Check sheet for the modelled part. Datum: model origin and axes. Units: mm. A direction names the side the tool comes from. Round coordinates to 2 decimals unless told otherwise and drop trailing zeros. Loops run counter-clockwise (first coordinate to the right, second up) from the corner with the lowest first, then second, coordinate; pieces in that order, holes last. Notation, with made-up numbers: (65, -24.75) -> (90, -24.75) arc R33 cw to (90, 7.25) -> close; hole circle Ø6 at (62, 41.5). An arc over 180 degrees is marked (long way). One line per question, with ' | ' between items.
```python
from build123d import *

# Parameters (mm, degrees)
SKETCH_1_R                   = 8
EXTRUDE_1_DEPTH              = 6
CUT_EXTRUDE_1_DEPTH          = 3.2
HOLE_WIZARD_M2_1_D           = 2.4
HOLE_WIZARD_M2_1_CBORE_D     = 4.2
HOLE_WIZARD_M2_1_CBORE_DEPTH = 2.5
PATTERN_CIRCULAR_1_COUNT     = 4
HOLE_WIZARD_M4_1_D           = 5


with BuildPart() as part:
    # ｽｹｯﾁ1 → ﾎﾞｽ - 押し出し1 (new body)
    with BuildSketch(Plane.XY):
        Circle(SKETCH_1_R)
    extrude(amount=EXTRUDE_1_DEPTH)

    # ｽｹｯﾁ2 → ｶｯﾄ - 押し出し1 (cut)
    with BuildSketch(Plane.XY.offset(6)):
        Polygon((4.070319398, 0), (2.035159699, 3.525), (-2.035159699, 3.525), (-4.070319398, 0), (-2.035159699, -3.525), (2.035159699, -3.525), align=None)
    extrude(amount=-CUT_EXTRUDE_1_DEPTH, mode=Mode.SUBTRACT)

    # M2 丸平ねじ用座ぐり穴1 (through all)
    with Locations(Plane(origin=(0, 0, 0), x_dir=(-1, 0, 0), z_dir=(0, 0, -1))):
        with Locations((6, 0)):
            hole_wizard_m2_1 = CounterBoreHole(HOLE_WIZARD_M2_1_D / 2, HOLE_WIZARD_M2_1_CBORE_D / 2, HOLE_WIZARD_M2_1_CBORE_DEPTH)

    # 円形ﾊﾟﾀｰﾝ1: M2 丸平ねじ用座ぐり穴1 ×4 about axis
    pattern_circular_1_axis = Axis((0, 0, 0), (0, 0, 1))
    for i in range(1, PATTERN_CIRCULAR_1_COUNT):
        add(hole_wizard_m2_1.rotate(pattern_circular_1_axis, i * 360 / PATTERN_CIRCULAR_1_COUNT), mode=Mode.SUBTRACT)

    # M4 すきま穴1 (through all)
    with Locations(Plane(origin=(0, 0, 0), x_dir=(-1, 0, 0), z_dir=(0, 0, -1))):
        with Locations((0, 0)):
            Hole(HOLE_WIZARD_M4_1_D / 2)


solid = part.part
```
(1) Sectioned sample at B-B, the plane y = 6. Record the cut outline in (x, z).
Answer:
outline: (-5.29, 0) -> (-2.1, 0) -> (-2.1, 2.5) -> (-1.2, 2.5) -> (-1.2, 6) -> (-5.29, 6) -> close; (1.2, 2.5) -> (2.1, 2.5) -> (2.1, 0) -> (5.29, 0) -> (5.29, 6) -> (1.2, 6) -> close
(2) Sectioned sample at C-C, the plane x = -1. Record the cut outline in (y, z) (3 decimals).
Answer:
outline: (-7.937, 0) -> (-7.847, 0) -> (-7.847, 2.5) -> (-6.663, 2.5) -> (-6.663, 6) -> (-7.937, 6) -> close; (-5.337, 2.5) -> (-4.153, 2.5) -> (-4.153, 0) -> (-2.291, 0) -> (-2.291, 2.8) -> (-3.525, 2.8) -> (-3.525, 6) -> (-5.337, 6) -> close; (2.291, 0) -> (4.153, 0) -> (4.153, 2.5) -> (5.337, 2.5) -> (5.337, 6) -> (3.525, 6) -> (3.525, 2.8) -> (2.291, 2.8) -> close; (6.663, 2.5) -> (7.847, 2.5) -> (7.847, 0) -> (7.937, 0) -> (7.937, 6) -> (6.663, 6) -> close
(3) Go/stop test with flat-tipped pins: pin 1 (2 mm diameter, centred on x = 1.5, z = 1.5, fed in from +Y); pin 2 (2 mm diameter, centred on x = 6, y = 0, fed in from +Z); pin 3 (4 mm diameter, centred on x = 0, y = 6, fed in from -Z); pin 4 (2 mm diameter, centred on x = -2, y = 0, fed in from +Z). Record where each tip stops, or that it passes through.
Answer:
pin 1: stops at y = 7.97 | pin 2: passes through | pin 3: stops at z = 2.5 | pin 4: stops at z = 2.8
(4) Sectioned sample at A-A, the plane z = 4.3. Record the cut outline in (x, y) (3 decimals).
Answer:
outline: circle Ø16 at (0, 0); hole circle Ø2.4 at (-6, 0); hole (-4.07, 0) -> (-2.035, -3.525) -> (2.035, -3.525) -> (4.07, 0) -> (2.035, 3.525) -> (-2.035, 3.525) -> close; hole circle Ø2.4 at (0, -6); hole circle Ø2.4 at (0, 6); hole circle Ø2.4 at (6, 0)
(5) Mould release check, pull along X, two halves, no side actions. Record for faces 4 (the face through (-0.05, -7.2, 4.27)), 5 (the face through (0, 4, 6)), 6 (the face through (7.39, -3.06, 2.96)): +X half, -X half, draft (parallel to the pull), parting line (faces both ways), or undercut.
Answer:
face 4: undercut | face 5: draft | face 6: parting line
(6) Set-up check for faces 1 (the face through (0.05, 7.2, 4.27)), 2 (the face through (-7, -1, 2.5)), 3 (the face through (3.067, 1.738, 4.422)): record each of +Z, -Z, +X, -X, +Y, -Y from which the full face is reachable in a straight line by a thin tool's end or side.
Answer:
face 1: +Z, -Z | face 2: -Z | face 3: +Z
(7) Scan lines: probe 1 along X at (y, z) = (0.75, 4.2); probe 2 along Y at (x, z) = (1.75, 1.15); probe 3 along Y at (x, z) = (0.25, 3.2) (3 decimals). Record each from-to range of solid material in increasing order.
Answer:
probe 1: x = -7.96 to -6.94, -5.06 to -3.64, 3.64 to 5.06, 6.94 to 7.96 | probe 2: y = -7.81 to -7.16, -4.84 to -1.79, 1.79 to 4.84, 7.16 to 7.81 | probe 3: y = -7.996 to -7.174, -4.826 to -3.525, 3.525 to 4.826, 7.174 to 7.996
